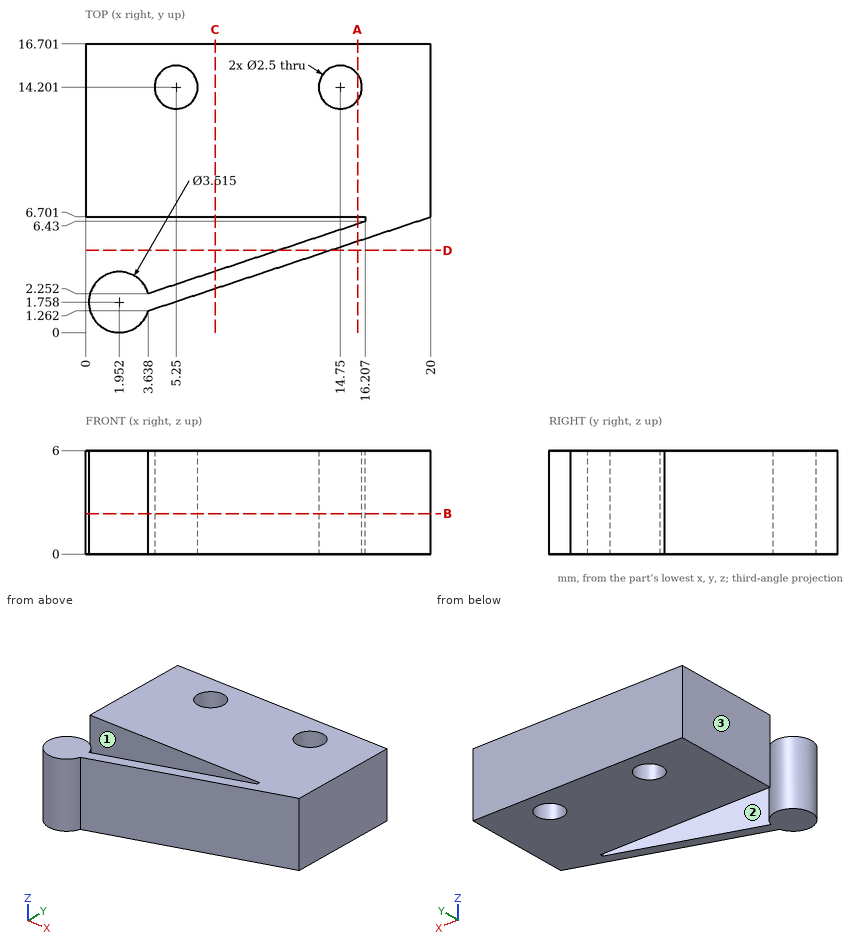
The figure shows three views and two pictorial views of one solid part (mm, origin at its lowest corner). Answer the questions. Coordinates: 2 decimals unless noted, no trailing zeros. Order: outer loops, then holes, each group sorted by start corner. A loop starts at its lowest first (then second) coordinate and runs counter-clockwise, first axis right, second up.
Q1. For a pull along X with two mould halves and no side action, classify the marked faces 1, 2 and 3 as pulls with the +X half, pulls with the -X half, needs draft (parallel to the pull), parting line crosses it, or undercut.
Q2. A cutting plane is placed at C-C, the plane x = 7.5. Write down the section's boundary in (y, z) (1 decimal).
Q3. A cutting plane is placed at D-D, the plane y = 4.75. Write down the section's boundary in (x, z).
Q4. Given P1, Ø4, axis at x = 14.75, y = 14.2, coming from the -Z side; P2, Ø3, axis at x = 10, z = 3.5, coming from the -Y side, each flat-ended and moving along its own axis, determine where each tip first touches the part or whether it passes through.
Q5. A cutting plane is placed at A-A, the plane x = 15.75. Write down the section's boundary in (y, z).
Q6. A cutting plane is placed at B-B, the plane z = 2.35. State how many separate pieces and enclosed holes the cut face has, and give its area (3 significant figures).
Q7. Consider line 1 (X direction, y = 14.25, z = 0.5); line 2 (Y direction, x = 5.25, z = 3.8); line 3 (Y direction, x = 7.25, z = 4.5). Determine where each line is inside the solid, lowest interval first.
Answers follow:
1. face 1: needs draft
1. face 2: undercut
1. face 3: pulls with the -X half
2. outline: (2.5, 0) - (3.5, 0) - (3.5, 6) - (2.5, 6) - close; (6.7, 0) - (16.7, 0) - (16.7, 6) - (6.7, 6) - close
3. outline: (11.15, 0) - (14.13, 0) - (14.13, 6) - (11.15, 6) - close
4. P1: stops at z = 0
4. P2: stops at y = 2.88
5. outline: (5.29, 0) - (6.28, 0) - (6.28, 6) - (5.29, 6) - close; (6.7, 0) - (13.45, 0) - (13.45, 6) - (6.7, 6) - close; (14.95, 0) - (16.7, 0) - (16.7, 6) - (14.95, 6) - close
6. separate pieces: 1
6. enclosed holes: 2
6. area: 215 mm2
7. line 1: x = 0 to 4, 6.5 to 13.5, 16 to 20
7. line 2: y = 1.8 to 2.79, 6.7 to 12.95, 15.45 to 16.7
7. line 3: y = 2.46 to 3.45, 6.7 to 16.7
